```python
from build123d import *

# Parameters (mm, degrees)
F1_DEPTH = 1.5
F3_W     = 3.4
F3_H     = 3.4
F3_W_2   = 2.5
F3_H_2   = 1.5
F4_DEPTH = 1.5
F5_W     = 3
F5_H     = 3
F5_W_2   = 2.042156
F5_H_2   = 2.253413
F5_W_3   = 1.8
F5_H_3   = 1
F5_W_4   = 2
F5_W_5   = 0.8
F5_H_4   = 1.5
F5_W_6   = 1.5
F5_H_5   = 0.8
F6_DEPTH = 1.5


with BuildPart() as f1:
    # F0 (on Top) → F1 (new body)
    with BuildSketch(Plane.XY):
        Polygon((-7, -14), (7, -14), (7, 11), (6.7, 11), (6.7, 14), (4.1, 14), (4.1, 11), (1.5, 11), (1.5, 14), (-1.5, 14), (-1.5, 11), (-4.1, 11), (-4.1, 14), (-6.7, 14), (-6.7, 11), (-7, 11), align=None)
    extrude(amount=F1_DEPTH)

    # F3 (on face) → F4 (join)
    with BuildSketch(Plane.XY.offset(1.5)):
        with Locations((-5, 8.8)):
            Rectangle(F3_W, F3_H)
        with Locations((-5, 4.8)):
            Rectangle(F3_W, F3_H)
        with Locations((-5, 0.8)):
            Rectangle(F3_W, F3_H)
        with Locations((-5, -3.2)):
            Rectangle(F3_W, F3_H)
        with Locations((0, 8.8)):
            Rectangle(F3_W, F3_H)
        with Locations((0, 4.8)):
            Rectangle(F3_W, F3_H)
        with Locations((0, 0.8)):
            Rectangle(F3_W, F3_H)
        with Locations((0, -3.2)):
            Rectangle(F3_W, F3_H)
        with Locations((5, 8.8)):
            Rectangle(F3_W, F3_H)
        with Locations((5, 4.8)):
            Rectangle(F3_W, F3_H)
        with Locations((5, 0.8)):
            Rectangle(F3_W, F3_H)
        with Locations((5, -3.2)):
            Rectangle(F3_W, F3_H)
        with Locations((-5.45, -6.65)):
            Rectangle(F3_W_2, F3_H_2)
        with Locations((-5.45, -8.7)):
            Rectangle(F3_W_2, F3_H_2)
        with Locations((-2.5, -6.65)):
            Rectangle(F3_W_2, F3_H_2)
        with Locations((-2.5, -8.7)):
            Rectangle(F3_W_2, F3_H_2)
        with Locations((0.45, -6.65)):
            Rectangle(F3_W_2, F3_H_2)
        with Locations((0.45, -8.7)):
            Rectangle(F3_W_2, F3_H_2)
        with Locations((-5.45, -10.75)):
            Rectangle(F3_W_2, F3_H_2)
        with Locations((-2.5, -10.75)):
            Rectangle(F3_W_2, F3_H_2)
    extrude(amount=F4_DEPTH)

    # F5 (on face) → F6 (join)
    with BuildSketch(Plane(origin=(0, 0, 0), x_dir=(1, 0, 0), z_dir=(0, 0, -1))):
        with Locations((2.570299, -3.256886)):
            Rectangle(F5_W, F5_H)
        with Locations((3.873054, 5.862395)):
            Rectangle(F5_W_2, F5_H_2)
        with Locations((-5.5, 10.5)):
            Rectangle(F5_W_3, F5_H)
        with Locations((-5.5, 6.813054)):
            Rectangle(F5_W_3, F5_H_3)
        with Locations((-5.6, 4.277964)):
            Rectangle(F5_W_4, F5_H_3)
        with Locations((-3.732216, 10.157964)):
            Rectangle(F5_W_5, F5_H_4)
        with Locations((-4.542036, 13.397247)):
            Rectangle(F5_W_6, F5_H_5)
    extrude(amount=F6_DEPTH)


solid = f1.part
```
Could you check a few things on this model? Use its own coordinates, in mm. A direction names the side the tool comes from. Round coordinates to 2 decimals unless told otherwise and drop trailing zeros. Loops run counter-clockwise (first coordinate to the right, second up) from the corner with the lowest first, then second, coordinate; pieces in that order, holes last.
Q1. Please list where these lines run through material, in increasing order: L1, parallel to Y at x = -4, z = 2.6; L2, parallel to X at y = 4.5, z = 2.05; L3, parallel to X at y = -8, z = 2.45.
Q2. On a 3-axis mill with a long thin cutter (end or side, diameter ignored), from which of +Z, -Z, +X, -X, +Y, -Y can I reach the whole of each face in a straight line? I mean faces 5 (the flat face through (4, -4.736, -1)), 6 (the flat face through (-5, -13.797, -1)), 7 (the flat face through (-5.292, -13.4, -0.7)), 8 (the flat face through (-1.7, 5, 2)), 9 (the flat face through (5, 10.5, 2)). Say none if no direction works.
Q3. For P1, Ø1.6, axis at x = -6, z = 2.5, coming from the +Y side; P2, Ø1, axis at x = 5, y = -2, coming from the -Z side; P3, Ø1.6, axis at y = -10.5, z = -1, coming from the +X side, each with a flat end and sliding along its axis, tell me the tip position at first contact or that it passes through.
Q4. I want a section at A-A (z = -0.8). Write out the boundary of the cut face in (x, y), and give its area (3 significant figures).
Q5. Thinking about a two-plate mould opening in Y: for faces 1 (the flat face through (-6.7, -7, 2)), 2 (the flat face through (-5, -12.997, -1)), 3 (the flat face through (-5, -11.5, 2)), 4 (the flat face through (0, 14, 1)), which applies, pulls with the +Y half, pulls with the -Y half, needs draft (parallel to the pull), parting line crosses it, or undercut?
Q6. I want a section at D-D (z = 1.95). Give the number of separate pieces and of enclosed holes in the cut face, and give its area (3 significant figures).
Q7. I want a section at C-C (x = 6). Write out the boundary of the cut face in (y, z), and give its area (3 significant figures).
Q8. I want a section at B-B (y = 3.5). Write out the boundary of the cut face in (x, z), and give its area (3 significant figures).
Answer below:
1. L1: y = -4.9 to -1.5, -0.9 to 2.5, 3.1 to 6.5, 7.1 to 10.5
1. L2: x = -6.7 to -3.3, -1.7 to 1.7, 3.3 to 6.7
1. L3: x = -6.7 to -4.2, -3.75 to -1.25, -0.8 to 1.7
2. face 5: -Z, +X
2. face 6: -Z, +X, -X, -Y
2. face 7: -Z, -X, -Y
2. face 8: +Z, +Y
2. face 9: +Z, +X, -X, +Y
3. P1: stops at y = 10.5
3. P2: stops at z = 0
3. P3: stops at x = -3.33
4. outline: (-6.6, -4.78) - (-4.6, -4.78) - (-4.6, -3.78) - (-6.6, -3.78) - close; (-6.4, -12) - (-4.6, -12) - (-4.6, -9) - (-6.4, -9) - close; (-6.4, -7.31) - (-4.6, -7.31) - (-4.6, -6.31) - (-6.4, -6.31) - close; (-5.29, -13.8) - (-3.79, -13.8) - (-3.79, -13) - (-5.29, -13) - close; (-4.13, -10.91) - (-3.33, -10.91) - (-3.33, -9.41) - (-4.13, -9.41) - close; (1.07, 1.76) - (4.07, 1.76) - (4.07, 4.76) - (1.07, 4.76) - close; (2.85, -6.99) - (4.89, -6.99) - (4.89, -4.74) - (2.85, -4.74) - close
4. area: 25.2 mm2
5. face 1: needs draft
5. face 2: undercut
5. face 3: pulls with the -Y half
5. face 4: pulls with the +Y half
6. separate pieces: 20
6. enclosed holes: 0
6. area: 169 mm2
7. outline: (-14, 0) - (14, 0) - (14, 1.5) - (10.5, 1.5) - (10.5, 3) - (7.1, 3) - (7.1, 1.5) - (6.5, 1.5) - (6.5, 3) - (3.1, 3) - (3.1, 1.5) - (2.5, 1.5) - (2.5, 3) - (-0.9, 3) - (-0.9, 1.5) - (-1.5, 1.5) - (-1.5, 3) - (-4.9, 3) - (-4.9, 1.5) - (-14, 1.5) - close
7. area: 62.4 mm2
8. outline: (-7, 0) - (1.07, 0) - (1.07, -1.5) - (4.07, -1.5) - (4.07, 0) - (7, 0) - (7, 1.5) - (6.7, 1.5) - (6.7, 3) - (3.3, 3) - (3.3, 1.5) - (1.7, 1.5) - (1.7, 3) - (-1.7, 3) - (-1.7, 1.5) - (-3.3, 1.5) - (-3.3, 3) - (-6.7, 3) - (-6.7, 1.5) - (-7, 1.5) - close
8. area: 40.8 mm2
